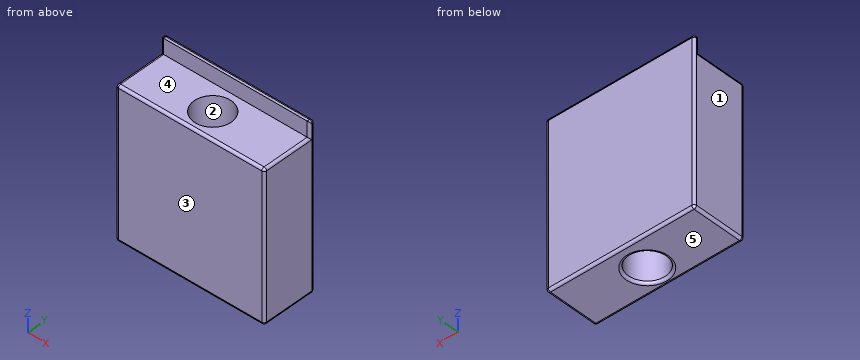
from build123d import *

# Parameters (mm, degrees)
F1_DEPTH = 60
F3_DEPTH = 60
F4_R     = 0.99999


# Not quite as in the source:
# - a fillet or chamfer is up to 0.001 mm smaller than in the source, because OpenCascade refuses the exact size
# - the program builds the solid bodies; features that only make, move or delete a surface that nothing else refers to are left out


with BuildPart() as f1:
    # F0 (on Top) → F1 (new body)
    with BuildSketch(Plane.XY):
        with BuildLine():
            Line((-60, 20), (-60, 10))
            Line((-60, 10), (-37.5, 10))
            ThreePointArc((-37.5, 10), (-35.3033008589, 15.3033008589), (-30, 17.5))
            Line((-30, 17.5), (-30, 20))
            Line((-30, 20), (-60, 20))
        make_face()
        with BuildLine():
            Line((-22.5, 10), (0, 10))
            Line((0, 10), (0, 20))
            Line((0, 20), (-30, 20))
            Line((-30, 20), (-30, 17.5))
            ThreePointArc((-30, 17.5), (-24.6966991411, 15.3033008589), (-22.5, 10))
        make_face()
        with BuildLine():
            Line((-30, 0), (0, 0))
            Line((0, 0), (0, 10))
            Line((0, 10), (-22.5, 10))
            ThreePointArc((-22.5, 10), (-24.6966991411, 4.6966991411), (-30, 2.5))
            Line((-30, 2.5), (-30, 0))
        make_face()
        with BuildLine():
            Line((-60, 0), (-30, 0))
            Line((-30, 0), (-30, 2.5))
            ThreePointArc((-30, 2.5), (-35.3033008589, 4.6966991411), (-37.5, 10))
            Line((-37.5, 10), (-60, 10))
            Line((-60, 10), (-60, 0))
        make_face()
    extrude(amount=F1_DEPTH)

    # F2 (on face) → F3 (join)
    with BuildSketch(Plane(origin=(-60, 0, 0), x_dir=(0, -1, 0), z_dir=(-1, 0, 0))):
        Polygon((-22, 0), (-20, 0), (-20, 60), (-20, 66.1894296401), (-22, 66.1894296401), align=None)
    extrude(amount=-F3_DEPTH)

    # F4 (radius 1 in the source; OpenCascade refuses exactly that, so slightly less here)
    f4_edges = [f1.edges().sort_by_distance(p)[0] for p in [
        (0, 22, 33.094715),
        (-60, 0, 30),
        (-60, 11, 0),
        (-60, 22, 33.094715),
        (-60, 21, 66.18943),
        (-60, 20, 63.094715),
        (-60, 10, 60),
        (-30, 22, 66.18943),
        (-30, 22, 0),
        (-30, 0, 0),
        (0, 11, 0),
        (-30, 17.5, 0),
        (0, 0, 30),
        (0, 10, 60),
        (0, 20, 63.094715),
        (0, 21, 66.18943),
        (-30, 0, 60),
    ]]
    fillet(f4_edges, radius=F4_R)


solid = f1.part
Read the model definition and answer for the solid it produces. Units are mm, in the model's axes. Face numbers are marked on the shaded views. A direction names the side the tool comes from. Give positions to 0.01 mm unless a question says otherwise; leave off trailing zeros. Loops run counter-clockwise (first coordinate to the right, second up) from the corner with the lowest first, then second, coordinate; pieces in that order, holes last. Notation, with made-up numbers: M 47,57 L 72,57 A18 ccw 72,71 Z; hole C 60.25,-7.5 d5. An arc over 180 degrees is marked long. Write each question's results on one line, items separated by ' | '.
1. Section B-B on x = -54 is taken. Give the vertices of the cut face in (y, z).
Values:
outline: M 0,1 A1 ccw 1,0 L 21,0 A1 ccw 22,1 L 22,65.19 A1 ccw 21,66.19 L 20,66.19 L 20,60 L 1,60 A1 ccw 0,59 Z
2. Given pin 1 (1.5 mm diameter, centred on x = -23.5, y = 18.5, fed in from +Z); pin 2 (1.9 mm diameter, centred on x = -19, z = 64, fed in from -Y), each flat-ended and moving along its own axis, determine where each tip first touches the part or whether it passes through.
Values:
pin 1: stops at z = 60 | pin 2: stops at y = 20
3. Straight lines are drawn through the part: line 1 (X direction, y = 9.75, z = 3.5); line 2 (Y direction, x = -30, z = 36); line 3 (Z direction, x = -16.5, y = 15). For each, find the intervals that lie inside material, in ascending order. Write a range as [from, to].
Values:
line 1: x = [-60, -37.5], [-22.5, 0] | line 2: y = [0, 2.5], [17.5, 22] | line 3: z = [0, 60]
4. A tool of negligible diameter and unlimited length cuts with its end or side. For the marked faces 4 and 5, from which of +Z, -Z, +X, -X, +Y, -Y can it reach the whole face along a straight path? Write none if from no direction.
Values:
face 4: +Z, +X, -X, -Y | face 5: -Z, +X, -X, +Y, -Y
5. Section A-A on z = 40.5 is taken. Give the vertices of the cut face in (x, y).
Values:
outline: M -60,1 A1 ccw -59,0 L -1,0 A1 ccw 0,1 L 0,21 A1 ccw -1,22 L -59,22 A1 ccw -60,21 Z; hole C -30,10 d15
6. The mould has two halves that part along Y. Classify the marked faces 1, 2 and 3: pulls with the +Y half, pulls with the -Y half, needs draft (parallel to the pull), parting line crosses it, or undercut.
Values:
face 1: needs draft | face 2: undercut | face 3: pulls with the -Y half
